Autodesk Inventor part; units mm, degrees
ref_plane "YZ Plane" through (0, 0, 0) normal (1, 0, 0) x (0, 1, 0)
ref_plane "XZ Plane" through (0, 0, 0) normal (0, 1, 0) x (-1, 0, 0)
ref_plane "XY Plane" through (0, 0, 0) normal (0, 0, 1) x (1, 0, 0)
sketch "Skizze1" plane through (0, 0, 0) normal (0, 0, 1) x (1, 0, 0)
  line L0 (0, 0) -> (40, 0)
  line L1 (40, 0) -> (40, 40)
  line L2 (40, 40) -> (0, 40)
  line L3 (0, 40) -> (0, 0)
  dimension "d0" = 40
  dimension "d1" = 40
extrude "Extrusion1" add sketch "Skizze1" along normal blind 2
sketch "Skizze3" plane through (0, 0, 2) normal (0, 0, 1) x (1, 0, 0)
  line L0 (0, 0) -> (0, 40)
  line L1 (40, 0) -> (0, 0)
  line L2 (40, 40) -> (40, 0)
  line L3 (0, 40) -> (40, 40)
  line L4 (36, 36) -> (36, 4)
  line L5 (36, 4) -> (4, 4)
  line L6 (4, 4) -> (4, 36)
  line L7 (4, 36) -> (36, 36)
  line L8 (38, 38) -> (38, 2)
  line L9 (38, 2) -> (2, 2)
  line L10 (2, 2) -> (2, 38)
  line L11 (2, 38) -> (38, 38)
  dimension "d14" = 4
  dimension "d15" = 2
hole "Bohrung2" at (38, 38, 2) at (2, 38, 2) at (2, 2, 2) at (38, 2, 2) direction (0, 0, -1) diameter 2.4 end through all
properties part number "13_0204_004-1"
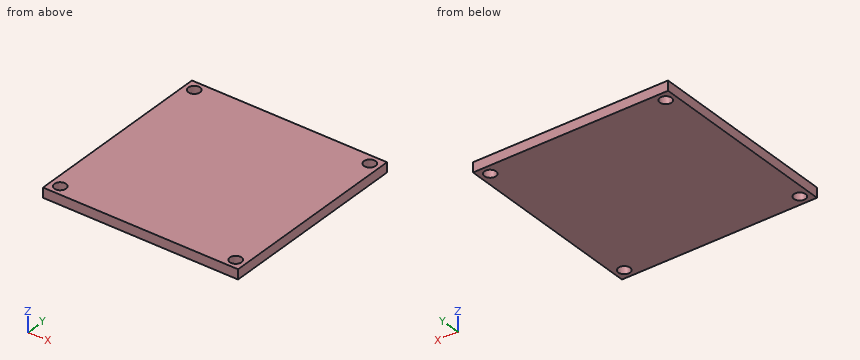
Part model, mm, in its own coordinate system. Give positions to 0.01 mm unless a question says otherwise; leave off trailing zeros. Order: outer loops, then holes, each group sorted by start corner. A loop starts at its lowest first (then second) coordinate and runs counter-clockwise, first axis right, second up. Notation, with made-up numbers: M 81.25,-2 L 126.25,-2 A32 ccw 126.25,24 Z; hole C 68,18 d2. An arc over 180 degrees is marked long. Use a Markdown table: item, result. Add a question column.
(1) Saw through at A-A, the plane y = 2. Give the cut face in (x, z), and give its area (3 significant figures).
(2) Probe line 1 along Y through (x, z) = (38, 1.5); line 2 along Y through (x, z) = (37, 0.45). List the from-to ranges inside material, lowest first. Write a range as [from, to].
Answer key:
| question | item | result |
|---|---|---|
| 1 | outline | M 0,0 L 0.8,0 L 0.8,2 L 0,2 Z; M 3.2,0 L 36.8,0 L 36.8,2 L 3.2,2 Z; M 39.2,0 L 40,0 L 40,2 L 39.2,2 Z |
| 1 | area | 70.4 mm^2 |
| 2 | line 1 | [0, 0.8], [3.2, 36.8], [39.2, 40] |
| 2 | line 2 | [0, 1.34], [2.66, 37.34], [38.66, 40] |
